Read the model definition and answer for the solid it produces. Units are mm, in the model's axes. A direction names the side the tool comes from. Round coordinates to 2 decimals unless told otherwise and drop trailing zeros. Order: outer loops, then holes, each group sorted by start corner. A loop starts at its lowest first (then second) coordinate and runs counter-clockwise, first axis right, second up. Notation, with made-up numbers: (18, 38.5) - (52, 38.5) arc R32 cw to (52, 69.5) - close; hole circle Ø9 at (9, 58). An arc over 180 degrees is marked (long way). Answer as a JSON object with one key per item and string values. Group by question number.
Q1. The mould has two halves that part along Y. Classify faces 1 (the flat face through (50, 0, 0)), 2 (the flat face through (1.7, 7.5, -51.2)), 3 (the cylindrical face through (92, 0, -1)): pulls with the +Y half, pulls with the -Y half, needs draft (parallel to the pull), parting line crosses it, or undercut.
Q2. A cutting plane is placed at A-A on y = 0. Determine the outline of the cut face in (x, z).
Q3. A cutting plane is placed at B-B on x = 94.5. Determine the outline of the cut face in (y, z).
Q4. A cutting plane is placed at C-C on z = -94.5. Determine the outline of the cut face in (x, y).
Q5. A cutting plane is placed at D-D on y = -5.25. Determine the outline of the cut face in (x, z), and give its area (3 significant figures).
Q6. Given pin 1 Ø4.5 at (x, y) = (47.5, 2.5) entering from -Z; pin 2 Ø1 at (y, z) = (2.5, -20.5) entering from +X, each flat-ended and moving along its own axis, determine where each tip first touches the part or whether it passes through.
Q7. Consider line 1 (Z direction, x = 1.45, y = 0); line 2 (X direction, y = 0, z = -0.55); line 3 (Z direction, x = 76.5, y = 5.5). Determine where each line is inside the solid, lowest interval first.
Q8. A tool of negligible diameter and unlimited length cuts with its end or side. For faces 4 (the flat face through (2, 0, -54)), 5 (the flat face through (0, 0, -52)), from which of +Z, -Z, +X, -X, +Y, -Y can it reach the whole face along a straight path? Write none if from no direction.
```python
from build123d import *

# Parameters (mm, degrees)
PAD_DEPTH            = 7.5
CYLINDER_R           = 2.5
CYLINDER_DEPTH       = 3
CYLINDER001_R        = 2.5
CYLINDER001_DEPTH    = 3
FILLET_R             = 4.95
BODY_PLACEMENT_ANGLE = 270


with BuildPart() as part:
    # Sketch → Pad (new body, symmetric)
    with BuildSketch(Plane.XY):
        Polygon((102, 0), (102, 2), (7, 2), (7, 7), (2, 7), (2, 102), (0, 102), (0, 0), align=None)
    extrude(amount=PAD_DEPTH, both=True)

    # Cylinder → Cylinder (cut)
    with BuildSketch(Plane(origin=(94.5, 3, 0), x_dir=(1, 0, 0), z_dir=(0, -1, 0))):
        Circle(CYLINDER_R)
    extrude(amount=CYLINDER_DEPTH, mode=Mode.SUBTRACT)

    # Cylinder001 → Cylinder001 (cut)
    with BuildSketch(Plane(origin=(0, 94.5, 0), x_dir=(0, 1, 0), z_dir=(1, 0, 0))):
        Circle(CYLINDER001_R)
    extrude(amount=CYLINDER001_DEPTH, mode=Mode.SUBTRACT)

    # Fillet
    fillet_edges = [part.edges().sort_by_distance(p)[0] for p in [
        (7, 7, 0),
    ]]
    fillet(fillet_edges, radius=FILLET_R)


with BuildPart() as part_1:
    # Body placement: moved
    add(part.part.rotate(Axis((0, 0, 0), (1, 0, 0)), BODY_PLACEMENT_ANGLE))


solid = part_1.part
```
Result set:
{
 "1": {"face 1": "needs draft", "face 2": "pulls with the +Y half", "face 3": "undercut"},
 "2": {"outline": "(0, -102) - (2, -102) - (2, -97) - (0, -97) - close; (0, -92) - (2, -92) - (2, -7) - (2.05, -7) arc R4.95 ccw to (7, -2.05) - (7, -2) - (92, -2) - (92, 0) - (0, 0) - close; (97, -2) - (102, -2) - (102, 0) - (97, 0) - close"},
 "3": {"outline": "(-7.5, -2) - (-2.5, -2) - (-2.5, 0) - (-7.5, 0) - close; (2.5, -2) - (7.5, -2) - (7.5, 0) - (2.5, 0) - close"},
 "4": {"outline": "(0, -7.5) - (2, -7.5) - (2, -2.5) - (0, -2.5) - close; (0, 2.5) - (2, 2.5) - (2, 7.5) - (0, 7.5) - close"},
 "5": {"outline": "(0, -102) - (2, -102) - (2, -7) - (2.05, -7) arc R4.95 ccw to (7, -2.05) - (7, -2) - (102, -2) - (102, 0) - (0, 0) - close", "area": "424 mm²"},
 "6": {"pin 1": "stops at z = -2", "pin 2": "stops at x = 2"},
 "7": {"line 1": "z = -102 to -97, -92 to 0", "line 2": "x = 0 to 92, 97 to 102", "line 3": "z = -2 to 0"},
 "8": {"face 4": "-Z, +X, +Y, -Y", "face 5": "+Z, -Z, -X, +Y, -Y"}
}
